Autodesk Inventor part; units mm, degrees
ref_plane "Work Plane1" through (0, 0, 0) normal (0.6427876, -0.7660444, 0) x (0, 0, -1)
ref_plane "Work Plane2" through (0, 14.3, -22) normal (0.6427876, 0.7660444, 0) x (0, 0, 1)
ref_plane "YZ Plane" through (0, 0, 0) normal (1, 0, 0) x (0, 1, 0)
sketch "Sketch1" plane through (0, 0, 0) normal (0, 1, 0) x (-1, 0, 0)
  circle A0 centre (0, 0) radius 5.075
  circle A1 centre (0, 0) radius 20
  line L0 (1.5, -3.825) -> (-1.5, -3.825)
  line L1 (-1.5, -3.825) -> (-1.5, -6.325)
  line L2 (-1.5, -6.325) -> (1.5, -6.325)
  line L3 (1.5, -6.325) -> (1.5, -3.825)
  line L4 (1.5, -3.825) -> (-1.5, -6.325) construction
  line L5 (-1.5, -3.825) -> (1.5, -6.325) construction
  circle A2 centre (0, 0) radius 2.5
  circle A3 centre (0, 0) radius 8.754
  point P0 (0, -5.075)
  point P1 (-1.5, -4.8483)
  point P2 (1.5, -4.8483)
  dimension "d0" = 10.15
  dimension "d1" = 40
  dimension "d2" = 1.25
  dimension "d3" = 3
  dimension "d17" = 5
extrude "Extrusion1" add sketch "Sketch1" along normal blind 14.3 contours A1 | A3
sketch "Sketch2" plane through (0, 0, 0) normal (1, 0, 0) x (0, 1, 0)
  line L0 (0, 0) -> (14.3, 0)
  line L1 (14.3, 0) -> (14.3, -22)
  line L2 (14.3, -22) -> (0, -22) construction
  line L3 (0, -22) -> (0, 0)
  line L4 (0, -22) -> (14.3, -22) construction
  line L5 (14.3, -22) -> (14.3, -20.0661)
  line L6 (0, -20) -> (14.3, -20)
  circle A0 centre (7.15, -22) radius 2.5
  line L7 (9.65, -22) -> (4.65, -22)
  line L8 (4.65, -22) -> (4.65, -30)
  line L9 (4.65, -30) -> (9.65, -30)
  line L10 (9.65, -30) -> (9.65, -22)
  line L11 (14.3, -20) -> (0, -20)
  line L12 (0, -20) -> (0, -30)
  line L13 (0, -30) -> (14.3, -30)
  line L14 (14.3, -30) -> (14.3, -20)
  point P0 (4.65, -30)
  point P1 (5.65, -20)
  point P2 (14.3, -22)
  point P3 (14.3, -20)
  point P4 (8.65, -20)
  point P5 (9.65, -30)
  point P6 (14.3, -20)
  point P7 (8.65, -20)
  dimension "d22" = 5
  dimension "d7" = 22
  dimension "d10" = 14.3
  dimension "d23" = 8
  dimension "d31" = 10
  dimension "d41" = 14.3
  dimension "d42" = 5
  dimension "d56" = 30
revolve "Revolution1" add sketch "Sketch2" angle 360 about axis through (0, 0, 0) along (0, 1, 0) contours L0 L1 L6 A0 L3 | L6 A0 L8 L13 L12 L3 | L1 L14 L13 L10 A0 L6 | A0 L6
extrude "Extrusion3" add sketch "Sketch1" against normal blind 2 contours A0 L3 L0 L1 | L1 L0 L3 A0 | A0 L3 L2 L1 | A3
revolve "Revolution4" cut sketch "Sketch2" angle 360 about axis through (0, 0, 0) along (0, 1, 0) contours A0 L6
sketch "Sketch3" plane through (0, 0, 0) normal (0, -1, 0) x (1, 0, 0)
  line L0 (0, 0) -> (0, -22)
  dimension "d25" = 22
ref_plane "Work Plane1" through (0, 0, 0) normal (0.6427876, -0.7660444, 0) x (0, 0, -1)
sketch "Sketch4" plane through (0, 0, 0) normal (0.6427876, -0.7660444, 0) x (0, 0, -1)
  ellipse E0 centre (0, 2.7318) end of major axis (22, 2.7318) minor radius 16.853
  line L0 (0, 0) -> (22, 0)
  circle A0 centre (22, 0) radius 3.75
  dimension "d27" = 22
  dimension "d28" = 7.5
extrude "Extrusion4" cut sketch "Sketch4" against normal blind 9 contours E0 L0 A0 | E0 A0 | E0 A0 L0 picked at (24.3646, -0.3075)
extrude "Extrusion5" cut sketch "Sketch4" along normal blind 7 contours E0 L0 A0 | E0 A0 | E0 A0 L0 picked at (24.3646, -0.3075)
ref_plane "Work Plane2" through (0, 14.3, -22) normal (0.6427876, 0.7660444, 0) x (0, 0, 1)
sketch "Sketch5" plane through (0, 14.3, -22) normal (0.6427876, 0.7660444, 0) x (0, 0, 1)
  ellipse E0 centre (22, -0.5142) end of major axis (27.075, -0.5142) minor radius 3.8877 (17.1517, -1.6633) -> (17.1517, 0.6348) ccw
  line L0 (22, -0.5142) -> (0, -0.5142)
  circle A0 centre (0, -0.5142) radius 3.75
  point P0 (22, 9.1919)
  dimension "d35" = 22
  dimension "d36" = 7.5
extrude "Extrusion6" cut sketch "Sketch5" against normal blind 9
extrude "Extrusion7" cut sketch "Sketch5" along normal blind 8
extrude "Extrusion8" cut sketch "Sketch1" along normal through all contours A0 L3 L0 L1 | L1 L0 L3 A0 | A0 L3 L2 L1 | A2
sketch "Sketch6" plane through (0, 14.3, 0) normal (0, 1, 0) x (1, 0, 0)
  circle A0 centre (0, 0) radius 15
  circle A1 centre (0, 0) radius 35.6972
  dimension "d45" = 30
extrude "Extrusion9" cut sketch "Sketch6" against normal blind 2.5
sketch "Sketch7" plane through (0, 0, 0) normal (0, -1, 0) x (1, 0, 0)
  circle A0 centre (0, 0) radius 2.5
  circle A1 centre (0, 0) radius 20
  line L0 (24, -7.5) -> (-24, -7.5)
  line L1 (-24, -7.5) -> (-24, 7.5)
  line L2 (-24, 7.5) -> (24, 7.5)
  line L3 (24, 7.5) -> (24, -7.5)
  line L4 (24, -7.5) -> (-24, 7.5) construction
  line L5 (-24, -7.5) -> (24, 7.5) construction
  circle A2 centre (0, 0) radius 11
  circle A3 centre (20, 0) radius 1.9
  circle A4 centre (-20, 0) radius 1.9
  dimension "d48" = 40
  dimension "d49" = 48
  dimension "d50" = 15
  dimension "d51" = 22
  dimension "d52" = 3.8
  dimension "d53" = 3.8
extrude "Extrusion10" cut sketch "Sketch7" against normal blind 4 contours A1 A3 | A1 A3 | A4 A1 | A1 A4
properties part number "spool_temp"
Verification items for the finished model (mm, model axes). A direction names the side the tool comes from. Give positions to 0.01 mm unless a question says otherwise; leave off trailing zeros. Order: outer loops, then holes, each group sorted by start corner. A loop starts at its lowest first (then second) coordinate and runs counter-clockwise, first axis right, second up. Notation, with made-up numbers: M 33,-14.75 L 69,-14.75 A15 ccw 69,-0.75 Z; hole C -36.75,54.5 d11. An arc over 180 degrees is marked long. Use one line per item in the form item = value. Start each with the question number.
Q1. Section check B-B (y = 0.75). Count the separate pieces of the cut face and the enclosed holes in it, then the cut area to 3 significant figures.
Q2. Section check A-A (x = 23.5). Enter the section's corners in (y, z), then the cut area to 3 significant figures.
Q3. Access from +Z, -Z, +X, -X, +Y, -Y to the whole of each face (thin tool, end or side, straight path). Record for faces 4 (the flat face through (6, 0, 7)), 5 (the flat face through (-18, 4.65, 13)), 6 (the flat face through (-5.96, 6.75, -18.43)), 7 (the flat face through (-2, 0, -2)), 8 (the flat face through (-2, -2, -2)).
Q4. Go/stop test with flat-tipped pins: pin 1 Ø1.2 at (y, z) = (6, -6) entering from -X; pin 2 Ø5 at (x, z) = (1, 1.5) entering from +Y; pin 3 Ø5 at (x, z) = (-20, 0) entering from -Y; pin 4 Ø4 at (x, z) = (0, 0) entering from -Y. Record where each tip stops, or that it passes through.
Q5. Mould release check, pull along Z, two halves, no side actions. Record for faces 1 (the flat face through (-18, 9.65, 13)), 2 (the cylindrical face through (-1.32, 10.74, 29.97)), 3 (the cylindrical face through (0.118, 3.803, -19.236)): +Z half, -Z half, draft (parallel to the pull), parting line (faces both ways), or undercut.
Q6. Section check C-C (x = -25). Enter the section's corners in (y, z).
Q7. Scan lines: line 1 along X through (y, z) = (3, 0) (3 decimals); line 2 along Z through (x, y) = (0, -1.4); line 3 along Y through (x, z) = (7, -23). Record each from-to range of solid material in increasing order. Write a range as [from, to].
Evaluation:
q1.separate_pieces = 1
q1.enclosed_holes = 4
q1.area = 2,660 mm2
q2.outline = M 0,-18.65 L 4.65,-18.65 L 4.65,18.65 L 0,18.65 Z; M 9.65,-18.65 L 11.8,-18.65 L 11.8,18.65 L 9.65,18.65 Z
q2.area = 254 mm2
q3.face_4 = -Y
q3.face_5 = none
q3.face_6 = -Z
q3.face_7 = +Y
q3.face_8 = +Z, -Z, +X, -X, -Y
q4.pin_1 = -19.33
q4.pin_2 = 0
q4.pin_3 = 0
q4.pin_4 = through
q5.face_1 = draft
q5.face_2 = parting line
q5.face_3 = undercut
q6.outline = M 0,-16.58 L 4.65,-16.58 L 4.65,16.58 L 0,16.58 Z; M 9.65,-16.58 L 11.8,-16.58 L 11.8,16.58 L 9.65,16.58 Z
q7.line_1 = [-30, -21.9], [-18.1, -5.075], [5.075, 18.1], [21.9, 30]
q7.line_2 = [-8.75, -2.5], [2.5, 8.75]
q7.line_3 = [0, 4.65], [9.65, 11.8]
